from build123d import *

# Parameters (mm, degrees)
CROQUIS1_W              = 42
CROQUIS1_H              = 42
SALIENTE_EXTRUIR1_DEPTH = 39
CHAFL_N2_SIZE           = 4
CHAFL_N3_SIZE           = 0.5
CROQUIS2_R              = 15
CORTAR_EXTRUIR2_DEPTH   = 0.5
CHAFL_N4_SIZE           = 1
CROQUIS3_R              = 11
CROQUIS3_R_2            = 4.75
SALIENTE_EXTRUIR2_DEPTH = 2.5
CROQUIS4_R              = 2.5
SALIENTE_EXTRUIR3_DEPTH = 20
CHAFL_N5_SIZE           = 0.25
CROQUIS5_W              = 26.553784045
CROQUIS5_H              = 10.322094095
CORTAR_EXTRUIR3_DEPTH   = 17.5
CROQUIS6_R              = 1.5
CORTAR_EXTRUIR4_DEPTH   = 12
MATRIZC1_COUNT          = 4
CROQUIS7_W              = 14
CROQUIS7_H              = 16.933623344
CORTAR_EXTRUIR5_DEPTH   = 2
MATRIZC2_COUNT          = 4
CORTAR_EXTRUIR6_DEPTH   = 0.1
MATRIZC3_COUNT          = 4
CROQUIS9_R              = 5
CORTAR_EXTRUIR7_DEPTH   = 3
SALIENTE_EXTRUIR4_START = 0.1
CROQUIS10_R             = 4.65
CROQUIS10_R_2           = 2.5
SALIENTE_EXTRUIR4_DEPTH = 0.1


with BuildPart() as part:
    # Croquis1 → Saliente-Extruir1 (new body)
    with BuildSketch(Plane.XY):
        Rectangle(CROQUIS1_W, CROQUIS1_H)
    extrude(amount=SALIENTE_EXTRUIR1_DEPTH)

    # Chaflán2
    chafl_n2_edges = [part.edges().sort_by_distance(p)[0] for p in [
        (21, -21, 19.5),
        (-21, -21, 19.5),
        (-21, 21, 19.5),
        (21, 21, 19.5),
    ]]
    chamfer(chafl_n2_edges, length=CHAFL_N2_SIZE)

    # Chaflán3
    chafl_n3_edges = [part.edges().sort_by_distance(p)[0] for p in [
        (21, 0, 0),
        (21, 0, 39),
        (0, -21, 0),
        (-21, 0, 0),
        (0, 21, 0),
        (-19, -19, 0),
        (-19, 19, 0),
        (19, 19, 0),
        (19, -19, 0),
        (0, -21, 39),
        (0, 21, 39),
        (-21, 0, 39),
        (-19, -19, 39),
        (-19, 19, 39),
        (19, 19, 39),
        (19, -19, 39),
    ]]
    chamfer(chafl_n3_edges, length=CHAFL_N3_SIZE)

    # Croquis2 → Cortar-Extruir2 (cut)
    with BuildSketch(Plane(origin=(0, 0, 0), x_dir=(-1, 0, 0), z_dir=(0, 0, -1))):
        Circle(CROQUIS2_R)
    extrude(amount=-CORTAR_EXTRUIR2_DEPTH, mode=Mode.SUBTRACT)

    # Chaflán4
    # the kernel refuses this chamfer: 1 mm, written as the material it adds along each edge
    with BuildSketch(Plane(origin=(0, 0, 0.5), x_dir=(-1, 0, 0), z_dir=(0, -1, 0))) as chafl_n4_piece_1_section:
        Polygon((15, CHAFL_N4_SIZE), (15 - CHAFL_N4_SIZE, 0), (15, 0), align=None)
    chafl_n4_piece_1 = revolve(axis=Axis((0, 0, 0.5), (0, 0, -1)), mode=Mode.PRIVATE)
    chafl_n4_piece_1 = split(chafl_n4_piece_1, bisect_by=Plane(origin=(14.259533629, 0, 0), z_dir=(0, 0, 1)), keep=Keep.TOP, mode=Mode.PRIVATE)
    add(chafl_n4_piece_1)

    # Croquis3 → Saliente-Extruir2 (add)
    with BuildSketch(Plane(origin=(0, 0, 0.5), x_dir=(-1, 0, 0), z_dir=(0, 0, -1))):
        Circle(CROQUIS3_R)
        Circle(CROQUIS3_R_2, mode=Mode.SUBTRACT)
    extrude(amount=SALIENTE_EXTRUIR2_DEPTH)

    # Croquis4 → Saliente-Extruir3 (add)
    with BuildSketch(Plane(origin=(0, 0, 0.5), x_dir=(-1, 0, 0), z_dir=(0, 0, -1))):
        Circle(CROQUIS4_R)
    extrude(amount=SALIENTE_EXTRUIR3_DEPTH)

    # Chaflán5
    chafl_n5_edges = [part.edges().sort_by_distance(p)[0] for p in [
        (2.5, 0, -19.5),
    ]]
    chamfer(chafl_n5_edges, length=CHAFL_N5_SIZE)

    # Croquis5 → Cortar-Extruir3 (cut)
    with BuildSketch(Plane(origin=(0, 0, -19.5), x_dir=(-1, 0, 0), z_dir=(0, 0, -1))):
        with Locations((-4.826169949, 7.161047048)):
            Rectangle(CROQUIS5_W, CROQUIS5_H)
    extrude(amount=-CORTAR_EXTRUIR3_DEPTH, mode=Mode.SUBTRACT)

    # Croquis6 → Cortar-Extruir4 (cut)
    with BuildSketch(Plane(origin=(0, 0, 0), x_dir=(-1, 0, 0), z_dir=(0, 0, -1))):
        with Locations((-15.35, 15.35)):
            Circle(CROQUIS6_R)
    cortar_extruir4 = extrude(amount=-CORTAR_EXTRUIR4_DEPTH, mode=Mode.SUBTRACT)

    # MatrizC1: Cortar-Extruir4 ×4 about axis
    matrizc1_axis = Axis((0, 0, 0), (0, 0, 1))
    for i in range(1, MATRIZC1_COUNT):
        add(cortar_extruir4.rotate(matrizc1_axis, i * 360 / MATRIZC1_COUNT), mode=Mode.SUBTRACT)

    # Croquis7 → Cortar-Extruir5 (cut)
    with BuildSketch(Plane(origin=(-19, -19, 0), x_dir=(0, 0, 1), z_dir=(-0.7071067811865487, -0.7071067811865465, 0))):
        with Locations((19.5, 0)):
            Rectangle(CROQUIS7_W, CROQUIS7_H)
    cortar_extruir5 = extrude(amount=-CORTAR_EXTRUIR5_DEPTH, mode=Mode.SUBTRACT)

    # MatrizC2: Cortar-Extruir5 ×4 about axis
    matrizc2_axis = Axis((0, 0, 0), (0, 0, 1))
    for i in range(1, MATRIZC2_COUNT):
        add(cortar_extruir5.rotate(matrizc2_axis, i * 360 / MATRIZC2_COUNT), mode=Mode.SUBTRACT)

    # Croquis8 → Cortar-Extruir6 (cut)
    with BuildSketch(Plane(origin=(0, 21, 0), x_dir=(1, 0, 0), z_dir=(0, 1, 0))):
        Polygon((-14.171572875, -12.5), (-14.171572875, -26.5), (-14.171572875, -28), (14.171572875, -28), (14.171572875, -26.5), (14.171572875, -12.5), (14.171572875, -11), (-14.171572875, -11), align=None)
    cortar_extruir6 = extrude(amount=-CORTAR_EXTRUIR6_DEPTH, mode=Mode.SUBTRACT)

    # MatrizC3: Cortar-Extruir6 ×4 about axis
    matrizc3_axis = Axis((0, 0, 0), (0, 0, 1))
    for i in range(1, MATRIZC3_COUNT):
        add(cortar_extruir6.rotate(matrizc3_axis, i * 360 / MATRIZC3_COUNT), mode=Mode.SUBTRACT)

    # Croquis9 → Cortar-Extruir7 (cut)
    with BuildSketch(Plane.XY.offset(39)):
        Circle(CROQUIS9_R)
    extrude(amount=-CORTAR_EXTRUIR7_DEPTH, mode=Mode.SUBTRACT)

    # Croquis10 → Saliente-Extruir4 (add)
    with BuildSketch(Plane.XY.offset(36).offset(SALIENTE_EXTRUIR4_START)):
        Circle(CROQUIS10_R)
        with Locations(Location((0, 0, 0), (0, 0, 53.130102354))):
            Circle(CROQUIS10_R_2, mode=Mode.SUBTRACT)
    extrude(amount=-SALIENTE_EXTRUIR4_DEPTH)


solid = part.part
The listing builds one solid part. Answer for the finished solid, in the listing's coordinates (mm). A direction names the side the tool comes from. Coordinates: 2 decimals unless noted, no trailing zeros. Loops run counter-clockwise (first coordinate to the right, second up) from the corner with the lowest first, then second, coordinate; pieces in that order, holes last. Notation, with made-up numbers: M 83,77.25 L 137,77.25 A6 cw 137,82.25 Z; hole C 76,-39.75 d7. An arc over 180 degrees is marked long. Answer in a Markdown table with one row per item.
1) Find section B-B (z = 21). Determine the outline of the cut face in (x, y), then the cut area to 3 significant figures.
Answers below:
| item | result |
|---|---|
| outline | M -21,-14.17 L -14.17,-21 L -14.17,-20.9 L 14.17,-20.9 L 14.17,-21 L 21,-14.17 L 20.9,-14.17 L 20.9,14.17 L 21,14.17 L 14.17,21 L 14.17,20.9 L -14.17,20.9 L -14.17,21 L -21,14.17 L -20.9,14.17 L -20.9,-14.17 Z |
| area | 1,660 mm^2 |
2) Find section A-A (z = 3). Determine the outline of the cut face in (x, y), then the cut area to 3 significant figures.
Answers below:
| item | result |
|---|---|
| outline | M -21,-17 L -17,-21 L 17,-21 L 21,-17 L 21,17 L 17,21 L -17,21 L -21,17 Z; hole C -15.35,-15.35 d3; hole C -15.35,15.35 d3; hole C 15.35,-15.35 d3; hole C 15.35,15.35 d3 |
| area | 1,700 mm^2 |
3) Given pin 1 (3 mm diameter, centred on x = -10, y = 7, fed in from -Z); pin 2 (3.5 mm diameter, centred on x = -16, y = -19, fed in from -Z); pin 3 (8.5 mm diameter, centred on y = -5.5, z = 18, fed in from +X), each flat-ended and moving along its own axis, determine where each tip first touches the part or whether it passes through.
Answers below:
| item | result |
|---|---|
| pin 1 | z = -2 |
| pin 2 | z = 0 |
| pin 3 | x = 20.9 |
4) Which of the six approach directions +Z, -Z, +X, -X, +Y, -Y give full straight-line access (tool end or side, diameter ignored) to faces 5 (the flat face through (18, -18, 12.5)), 6 (the cylindrical face through (0.54, -2.44, -9.24)), 7 (the flat face through (-19, -19, 6))?
Answers below:
| item | result |
|---|---|
| face 5 | +X, -Y |
| face 6 | -Z |
| face 7 | +Z, -Z, -X, -Y |
5) Find section C-C (x = 18). Determine the outline of the cut face in (y, z), then the cut area to 3 significant figures.
Answers below:
| item | result |
|---|---|
| outline | M -20,0.5 L -19.29,0 L 19.29,0 L 20,0.5 L 20,12.5 L 17.17,12.5 L 17.17,26.5 L 20,26.5 L 20,38.5 L 19.29,39 L -19.29,39 L -20,38.5 L -20,26.5 L -17.17,26.5 L -17.17,12.5 L -20,12.5 Z |
| area | 1,480 mm^2 |
6) Find the intervals of material crossed by probe 1 along X at (y, z) = (15, 9); probe 2 along Y at (x, z) = (0, -1); probe 3 along Y at (x, z) = (-16.5, 8), in increasing order.
Answers below:
| item | result |
|---|---|
| probe 1 | -21 to -16.81, -13.89 to 13.89, 16.81 to 21 |
| probe 2 | -11 to -4.75, -2.5 to 2.5, 4.75 to 11 |
| probe 3 | -21 to -16.31, -14.39 to 14.39, 16.31 to 21 |
7) Determine the mould class of faces 1 (the cylindrical face through (-1.08, -4.88, 37.52)), 2 (the flat face through (17.63, 17.54, 19.4)), 3 (the flat face through (-15, 15, 12)), 4 (the flat face through (18, 18, 12.5)) for opening direction Y: released by +Y, released by -Y, zero draft, split by the parting line, or undercut.
Answers below:
| item | result |
|---|---|
| face 1 | undercut |
| face 2 | released by +Y |
| face 3 | undercut |
| face 4 | zero draft |
8) Find section D-D (y = -15.35). Determine the outline of the cut face in (x, z), then the cut area to 3 significant figures.
Answers below:
| item | result |
|---|---|
| outline | M -21,0.5 L -20.5,0 L -16.85,0 L -16.85,12 L -13.85,12 L -13.85,0 L 13.85,0 L 13.85,12 L 16.85,12 L 16.85,0 L 20.5,0 L 21,0.5 L 21,12.5 L 19.82,12.5 L 19.82,26.5 L 21,26.5 L 21,38.5 L 20.5,39 L -20.5,39 L -21,38.5 L -21,26.5 L -19.82,26.5 L -19.82,12.5 L -21,12.5 Z |
| area | 1,530 mm^2 |
